Autodesk Inventor part; units mm, degrees
ref_plane "YZ Plane" through (0, 0, 0) normal (1, 0, 0) x (0, 1, 0)
ref_plane "XZ Plane" through (0, 0, 0) normal (0, 1, 0) x (-1, 0, 0)
ref_plane "XY Plane" through (0, 0, 0) normal (0, 0, 1) x (1, 0, 0)
sketch "Sketch1" plane through (0, 0, 0) normal (0, 0, 1) x (1, 0, 0)
  circle A0 centre (0, 0) radius 76.2 construction
  circle A1 centre (0, 0) radius 7.1437
  circle A2 centre (0, 0) radius 12.7 construction
  circle A3 centre (0, 0) radius 19.05
  line L0 (0, 76.2) -> (0, 0) construction
  line L1 (0, 76.2) -> (4.2947, 60.1719)
  line L2 (4.2947, 60.1719) -> (-17.6011, 7.2873)
  circle A4 centre (0, 0) radius 60.325 construction
  arc A5 (27.9352, 66.3249) -> (0, 76.2) centre (0, 31.75) ccw
  line L3 (27.9352, 66.3249) -> (18.8874, -2.4836)
  circle A6 centre (0, 0) radius 45.2437 construction
  line L4 (34.9112, -28.7786) -> (0, 0) construction
  line L5 (34.9112, -28.7786) -> (25.7494, -23.595)
  line L6 (25.7494, -23.595) -> (18.4479, 4.7518)
  circle A7 centre (0, 0) radius 34.925 construction
  arc A8 (-42.6486, -15.1027) -> (34.9112, -28.7786) centre (0, 0) ccw
  line L7 (-42.6486, -15.1027) -> (-13.3288, 13.6105)
  line L8 (-42.6486, -15.1027) -> (0, 0) construction
  line L9 (-4.3483, 18.5471) -> (12.7964, 59.9565)
  line L10 (13.0349, 13.8922) -> (18.8778, 58.328)
  arc A9 (18.8778, 58.328) -> (12.7964, 59.9565) centre (15.7299, 58.7419) ccw
  line L11 (-10.5232, 7.11) -> (0, 0) construction
  line L12 (0, 0) -> (-4.542, 11.86) construction
  circle A10 centre (-4.542, 11.86) radius 1.7526
  circle A11 centre (-12.5421, 1.9966) radius 1.7526
  circle A12 centre (-8.0001, -9.8635) radius 1.7526
  circle A13 centre (4.542, -11.86) radius 1.7526
  circle A14 centre (12.5421, -1.9966) radius 1.7526
  circle A15 centre (8.0001, 9.8635) radius 1.7526
  point P0 (19.3687, 1.1767)
  point P1 (-15.8759, 11.4541)
  point P2 (-16.1113, 10.8856)
  dimension "d0" = 152.4
  dimension "d14" = 15.875
  dimension "d17" = 69.85
  dimension "d1" = 14.2875
  dimension "d2" = 25.4
  dimension "d8" = 38.1
  dimension "d9" = 15
  dimension "d11" = 44.45
  dimension "d12" = 15
  dimension "d15" = 90.4875
  dimension "d16" = 10
  dimension "d18" = 50.5
  dimension "d19" = 121
  dimension "d28" = 7.9375
  dimension "d29" = 7.9375
  dimension "d30" = 3.175
  dimension "d31" = 35
  dimension "d32" = 3.5052
  dimension "d35" = 360
extrude "Extrusion1" add sketch "Sketch1" along normal blind 6.35 contours A3 | A3 L6 L3 | A3 L10 A9 L9 L7 L2 L1 A5 L3 L6 | L3 L6 L5 A8 L7 L2 A3 | L2 L7 A3
fillet "Fillet1" radius 4.7625 6 edges at (19.3687, 1.1767, 3.175) (25.7494, -23.595, 3.175) (4.2947, 60.1719, 3.175) (-4.3483, 18.5471, 3.175) (13.0349, 13.8922, 3.175) (-16.1113, 10.8856, 3.175)
fillet "Fillet3" radius 3.175 1 edges at (-42.6486, -15.1027, 3.175)
sketch "Sketch2" plane through (0, 0, 6.35) normal (0, 0, 1) x (1, 0, 0)
  arc A0 (27.9352, 66.3249) -> (0, 76.2) centre (0, 31.75) ccw construction
  circle A1 centre (0, 0) radius 76.2 construction
equation "\"d29\" = d28"
properties part number "Blade" material "Steel, Alloy"
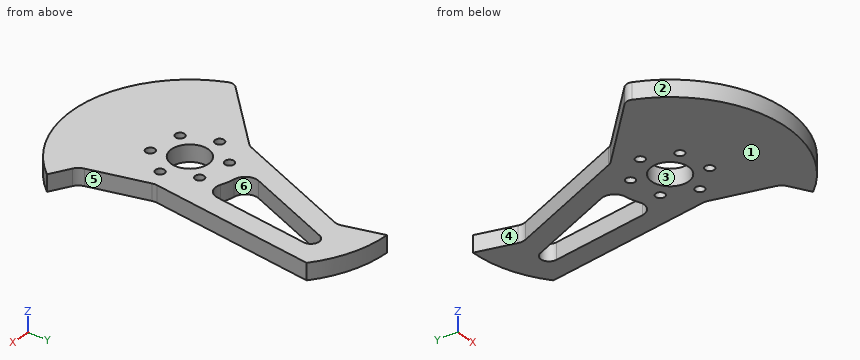
Geometry: final body of the model. Coordinates: model frame, mm. Face numbers are marked on the shaded views. A direction names the side the tool comes from. Round coordinates to 2 decimals unless told otherwise and drop trailing zeros. Loops run counter-clockwise (first coordinate to the right, second up) from the corner with the lowest first, then second, coordinate; pieces in that order, holes last. Notation, with made-up numbers: M -37,55.25 L 4,55.25 A14 ccw 4,73.25 Z; hole C 34.25,-17 d5. An arc over 180 degrees is marked long. Put each result on its own line as item: value. Start each with the question number.
(1) Section query A-A (z = 4.75). State how many separate pieces and enclosed holes the cut face has, then the cut area to 3 significant figures.
(2) Section query B-B (x = 29.5). Return loops of the section in (y, z), then the cut area to 3 significant figures.
(3) Set-up query: the marked faces 4, 5 and 6. Return all of +Z, -Z, +X, -X, +Y, -Y with unobstructed straight access to the full face (end or side cutting, diameter ignored); none if empty.
(4) Contact query for flat-ended pins moving along their axis: pin 1 Ø2 at (x, y) = (8, 9.86) entering from -Z; pin 2 Ø2 at (y, z) = (11, 4) entering from +X; pin 3 Ø2 at (y, z) = (34, 2) entering from -X; pin 4 Ø1.5 at (x, z) = (-13, 4) entering from -Y. Output: stop coordinate, or through.
(5) Section query C-C (x = -18). Return loops of the section in (y, z), then the cut area to 3 significant figures.
(6) Draft query along Y for the marked faces 1, 2 and 3. Return one class per face: +Y half, -Y half, draft (parallel to the pull), parting line (faces both ways), or undercut.
(7) Material intervals for line 1 along X through (y, z) = (-10.5, 2); line 2 along X through (y, z) = (29, 1.25); line 3 along X through (y, z) = (-3.5, 1.75), sorted ascending. Write a range as [from, to].
Findings below:
1. separate pieces: 1
1. enclosed holes: 8
1. area: 4,080 mm2
2. outline: M -34.3,0 L -25.72,0 L -25.72,6.35 L -34.3,6.35 Z
2. area: 54.5 mm2
3. face 4: +Z, -Z, -X
3. face 5: +Z, -Z, +X
3. face 6: +Z, -Z
4. pin 1: passes through
4. pin 2: stops at x = 20.79
4. pin 3: stops at x = -6.96
4. pin 4: stops at y = -43.55
5. outline: M -41.51,0 L 9.04,0 L 9.04,6.35 L -41.51,6.35 Z
5. area: 321 mm2
6. face 1: draft
6. face 2: -Y half
6. face 3: undercut
7. line 1: x = [-37.95, -9.63], [-6.37, 3.44], [5.65, 22.38]
7. line 2: x = [-8.61, -0.02], [15.02, 23.03]
7. line 3: x = [-30.8, -6.23], [6.23, 11.64], [13.44, 20.57]
